Can you work these out from the model? Positions are in its coordinate system, mm. Face numbers are marked on the shaded views. A direction names the side the tool comes from. Give positions to 0.01 mm unless a question says otherwise; leave off trailing zeros. Loops run counter-clockwise (first coordinate to the right, second up) from the corner with the lowest first, then second, coordinate; pieces in that order, holes last. Notation, with made-up numbers: (-33.75, -25.75) -> (-16.75, -25.75) arc R21 ccw to (-16.75, 4.25) -> close; hole circle Ø4 at (25, 2). An arc over 180 degrees is marked (long way). One line per question, with ' | ' between items.
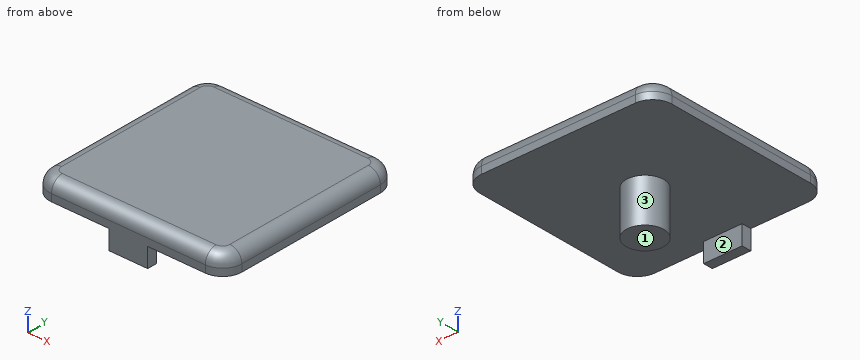
Autodesk Inventor part; units mm, degrees
ref_plane "YZ Plane" through (0, 0, 0) normal (1, 0, 0) x (0, 1, 0)
ref_plane "XZ Plane" through (0, 0, 0) normal (0, 1, 0) x (-1, 0, 0)
ref_plane "XY Plane" through (0, 0, 0) normal (0, 0, 1) x (1, 0, 0)
sketch "Sketch1" plane through (0, 0, 0) normal (0, 0, 1) x (1, 0, 0)
  line L0 (-20, 20) -> (20, 20)
  line L1 (20, 20) -> (20, -20)
  line L2 (20, -20) -> (-20, -20)
  line L3 (-20, -20) -> (-20, 20)
  point P0 (0, 0)
  point P1 (-20, 0)
  point P2 (0, 20)
  dimension "DimA" = 40
  dimension "DimB" = 40
extrude "Rectangluar End Cap" add sketch "Sketch1" along normal blind 4
sketch "Sketch6" plane through (0, 0, 4) normal (0, 0, 1) x (1, 0, 0)
  line L0 (-20, -20) -> (-20, 20) construction
  line L1 (20, -20) -> (-20, -20) construction
  circle A0 centre (0, 0) radius 3.9
  dimension "d37" = 20
  dimension "d38" = 20
  dimension "d39" = 7.8
extrude "Standard Post" add sketch "Sketch6" against normal blind 13
hole "Secure End Cap" [suppressed]
pattern_of_one "Rectangular Pattern3"
sketch "Sketch7" plane through (0, 0, 0) normal (0, 0, -1) x (-1, 0, 0)
  line L0 (-20, -20) -> (20, -20) construction
  line L1 (-4, -20) -> (4, -20)
  line L2 (4, -20) -> (4, -18)
  line L3 (4, -18) -> (-4, -18)
  line L4 (-4, -18) -> (-4, -20)
  line L5 (0, -18) -> (0, -20) construction
  point P0 (0, 0)
  dimension "d55" = 2
  dimension "d56" = 8
extrude "40x40 Orientation Tab" add sketch "Sketch7" along normal blind 4
fillet "Fillet5" radius 4 4 edges at (20, 20, 2) (-20, 20, 2) (-20, -20, 2) (20, -20, 2)
fillet "Fillet6" radius 2.5 8 edges at (-18.8284, -18.8284, 4) (0, -20, 4) (18.8284, -18.8284, 4) (20, 0, 4) (18.8284, 18.8284, 4) (0, 20, 4) (-18.8284, 18.8284, 4) (-20, 0, 4)
properties part number "18-813" material "Glass Filled Nylon"
Q1. If I drill on probe 1 along Z at (x, y) = (5.5, 0.5); probe 2 along Y at (x, z) = (-0.5, -3.5); probe 3 along X at (y, z) = (14, 2.25), over which ranges is the centre line in solid material (lowest first)? Write a range as from..to.
Entries:
probe 1: 0..4 | probe 2: -20..-18, -3.87..3.87 | probe 3: -19.88..19.88
Q2. If we section it at A-A (y = 0): Write out the boundary of the cut face in (x, z), plus the area to 3 significant figures.
Entries:
outline: (-20, 0) -> (-3.9, 0) -> (-3.9, -9) -> (3.9, -9) -> (3.9, 0) -> (20, 0) -> (20, 1.5) arc R2.5 ccw to (17.5, 4) -> (-17.5, 4) arc R2.5 ccw to (-20, 1.5) -> close | area: 228 mm²
Q3. For pin 1 Ø4.5 at (x, z) = (-1, -2.5) entering from +Y; pin 2 Ø1.5 at (x, y) = (-10.5, -0.5) entering from -Z; pin 3 Ø1.6 at (x, y) = (0, -18.5) entering from -Z; pin 4 Ø2 at (x, z) = (6.5, -2.5) entering from -Y, each with a flat end and sliding along its axis, tell me the tip position at first contact or that it passes through.
Entries:
pin 1: y = 3.9 | pin 2: z = 0 | pin 3: z = -4 | pin 4: through
Q4. If we section it at B-B (x = 0): Write out the boundary of the cut face in (y, z).
Entries:
outline: (-20, -4) -> (-18, -4) -> (-18, 0) -> (-3.9, 0) -> (-3.9, -9) -> (3.9, -9) -> (3.9, 0) -> (20, 0) -> (20, 1.5) arc R2.5 ccw to (17.5, 4) -> (-17.5, 4) arc R2.5 ccw to (-20, 1.5) -> close
Q5. If we section it at D-D (z = -6.75): Write out the boundary of the cut face in (x, y), plus the area to 3 significant figures.
Entries:
outline: circle Ø7.8 at (0, 0) | area: 47.8 mm²
Q6. On a 3-axis mill with a long thin cutter (end or side, diameter ignored), from which of +Z, -Z, +X, -X, +Y, -Y can I reach the whole of each face in a straight line? I mean the marked faces 1, 2 and 3. Say none if no direction works.
Entries:
face 1: -Z, +X, -X, +Y, -Y | face 2: -Z, +X, -X | face 3: -Z
Q7. If we section it at C-C (z = -1.5): Write out the boundary of the cut face in (x, y).
Entries:
outline: (-4, -20) -> (4, -20) -> (4, -18) -> (-4, -18) -> close; circle Ø7.8 at (0, 0)
